```python
from build123d import *

# Parameters (mm, degrees)
SKETCH1_W           = 25
SKETCH1_H           = 5
SKETCH2_R           = 3.625
BOSS_EXTRUDE1_DEPTH = 3
CUT_EXTRUDE1_DEPTH  = 37.463627082
CUT_EXTRUDE2_DEPTH  = 36.924867432
CUT_EXTRUDE3_DEPTH  = 36.924867432
CUT_EXTRUDE4_DEPTH  = 36.924867432
CUT_EXTRUDE5_DEPTH  = 36.924867432
CUT_EXTRUDE6_DEPTH  = 36.924867432
CUT_EXTRUDE7_DEPTH  = 36.924867432
CUT_EXTRUDE8_DEPTH  = 36.924867432
CUT_EXTRUDE9_DEPTH  = 37.463627082


with BuildPart() as part:
    # Sketch1 → Revolve1 (revolve)
    with BuildSketch(Plane(origin=(0, 0, 0), x_dir=(1, 0, 0), z_dir=(0, 1, 0))):
        with Locations((12.19, 88.3)):
            Rectangle(SKETCH1_W, SKETCH1_H)
    revolve(axis=Axis((-0.31, 0, -90.8), (0, 0, 1)))

    # Sketch2 → Boss-Extrude1 (add)
    with BuildSketch(Plane.XY.offset(-85.8)):
        with Locations((-0.31, 0)):
            Circle(SKETCH2_R)
    extrude(amount=BOSS_EXTRUDE1_DEPTH)

    # Sketch3 → Cut-Extrude1 (cut, through all)
    with BuildSketch(Plane(origin=(0, 0, -90.8), x_dir=(-1, 0, 0), z_dir=(0, 0, -1))):
        with BuildLine():
            Line((-1.738954013, -1.834199404), (2.358954013, -1.834199404))
            ThreePointArc((2.358954013, -1.834199404), (3.06, 0), (2.358954013, 1.834199404))
            Line((2.358954013, 1.834199404), (-1.738954013, 1.834199404))
            ThreePointArc((-1.738954013, 1.834199404), (-2.44, 0), (-1.738954013, -1.834199404))
        make_face()
    extrude(amount=-CUT_EXTRUDE1_DEPTH, mode=Mode.SUBTRACT)

    # Sketch4 → Cut-Extrude2 (cut, through all)
    with BuildSketch(Plane.XY.offset(-85.8)):
        with BuildLine():
            Line((5.725533906, 1), (15.382388155, 1))
            ThreePointArc((15.382388155, 1), (20.463725584, 8.604758878), (11.493300859, 10.389087297))
            Line((11.493300859, 10.389087297), (4.664873734, 3.560660172))
            ThreePointArc((4.664873734, 3.560660172), (4.339714607, 1.925974851), (5.725533906, 1))
        make_face()
    extrude(amount=-CUT_EXTRUDE2_DEPTH, mode=Mode.SUBTRACT)

    # Sketch5 → Cut-Extrude3 (cut, through all)
    with BuildSketch(Plane.XY.offset(-85.8)):
        with BuildLine():
            Line((-12.113300859, -10.389087297), (-5.284873734, -3.560660172))
            ThreePointArc((-5.284873734, -3.560660172), (-4.959714607, -1.925974851), (-6.345533906, -1))
            Line((-6.345533906, -1), (-16.002388155, -1))
            ThreePointArc((-16.002388155, -1), (-21.083725584, -8.604758878), (-12.113300859, -10.389087297))
        make_face()
    extrude(amount=-CUT_EXTRUDE3_DEPTH, mode=Mode.SUBTRACT)

    # Sketch6 → Cut-Extrude4 (cut, through all)
    with BuildSketch(Plane.XY.offset(-85.8)):
        with BuildLine():
            Line((3.250660172, 4.974873734), (10.079087297, 11.803300859))
            ThreePointArc((10.079087297, 11.803300859), (8.294758878, 20.773725584), (0.69, 15.692388155))
            Line((0.69, 15.692388155), (0.69, 6.035533906))
            ThreePointArc((0.69, 6.035533906), (1.615974851, 4.649714607), (3.250660172, 4.974873734))
        make_face()
    extrude(amount=-CUT_EXTRUDE4_DEPTH, mode=Mode.SUBTRACT)

    # Sketch7 → Cut-Extrude5 (cut, through all)
    with BuildSketch(Plane.XY.offset(-85.8)):
        with BuildLine():
            Line((-3.870660172, -4.974873734), (-10.699087297, -11.803300859))
            ThreePointArc((-10.699087297, -11.803300859), (-8.914758878, -20.773725584), (-1.31, -15.692388155))
            Line((-1.31, -15.692388155), (-1.31, -6.035533906))
            ThreePointArc((-1.31, -6.035533906), (-2.235974851, -4.649714607), (-3.870660172, -4.974873734))
        make_face()
    extrude(amount=-CUT_EXTRUDE5_DEPTH, mode=Mode.SUBTRACT)

    # Sketch8 → Cut-Extrude6 (cut, through all)
    with BuildSketch(Plane.XY.offset(-85.8)):
        with BuildLine():
            Line((15.382388155, -1), (5.725533906, -1))
            ThreePointArc((5.725533906, -1), (4.339714607, -1.925974851), (4.664873734, -3.560660172))
            Line((4.664873734, -3.560660172), (11.493300859, -10.389087297))
            ThreePointArc((11.493300859, -10.389087297), (20.463725584, -8.604758878), (15.382388155, -1))
        make_face()
    extrude(amount=-CUT_EXTRUDE6_DEPTH, mode=Mode.SUBTRACT)

    # Sketch9 → Cut-Extrude7 (cut, through all)
    with BuildSketch(Plane.XY.offset(-85.8)):
        with BuildLine():
            Line((-16.002388155, 1), (-6.345533906, 1))
            ThreePointArc((-6.345533906, 1), (-4.959714607, 1.925974851), (-5.284873734, 3.560660172))
            Line((-5.284873734, 3.560660172), (-12.113300859, 10.389087297))
            ThreePointArc((-12.113300859, 10.389087297), (-21.083725584, 8.604758878), (-16.002388155, 1))
        make_face()
    extrude(amount=-CUT_EXTRUDE7_DEPTH, mode=Mode.SUBTRACT)

    # Sketch10 → Cut-Extrude8 (cut, through all)
    with BuildSketch(Plane.XY.offset(-85.8)):
        with BuildLine():
            Line((-1.31, 6.035533906), (-1.31, 15.692388155))
            ThreePointArc((-1.31, 15.692388155), (-8.914758878, 20.773725584), (-10.699087297, 11.803300859))
            Line((-10.699087297, 11.803300859), (-3.870660172, 4.974873734))
            ThreePointArc((-3.870660172, 4.974873734), (-2.235974851, 4.649714607), (-1.31, 6.035533906))
        make_face()
    extrude(amount=-CUT_EXTRUDE8_DEPTH, mode=Mode.SUBTRACT)

    # Sketch11 → Cut-Extrude9 (cut, through all)
    with BuildSketch(Plane(origin=(0, 0, -90.8), x_dir=(-1, 0, 0), z_dir=(0, 0, -1))):
        with BuildLine():
            Line((-0.69, -15.692388155), (-0.69, -6.035533906))
            ThreePointArc((-0.69, -6.035533906), (-1.615974851, -4.649714607), (-3.250660172, -4.974873734))
            Line((-3.250660172, -4.974873734), (-10.079087297, -11.803300859))
            ThreePointArc((-10.079087297, -11.803300859), (-8.294758878, -20.773725584), (-0.69, -15.692388155))
        make_face()
    extrude(amount=-CUT_EXTRUDE9_DEPTH, mode=Mode.SUBTRACT)


solid = part.part
```
Could you check a few things on this model? Use its own coordinates, in mm. Round coordinates to 2 decimals unless told otherwise and drop trailing zeros. Loops run counter-clockwise (first coordinate to the right, second up) from the corner with the lowest first, then second, coordinate; pieces in that order, holes last. Notation, with made-up numbers: (84.5, -34.5) - (103.5, -34.5) arc R24 cw to (103.5, -14.5) - close; hole circle Ø8 at (33.5, 70). An arc over 180 degrees is marked (long way). Use CSV: the item, a comma, the result in double quotes.
Item 1: I need wall thicknesses on L1, parallel to Y at x = -20, z = -87.5; L2, parallel to Y at x = -6.81, z = -87.6; L3, parallel to X at y = 6.5, z = -87. Which ranges of each line are inside material? Lowest first, please. Write a range as [from, to].
Here are the results:
L1,"y = [-15.4, -10.28], [-2.72, 2.72], [10.28, 15.4]"
L2,"y = [-24.14, -21.19], [-7.91, -5.09], [-1, 1], [5.09, 7.91], [21.19, 24.14]"
L3,"x = [-24.45, -21.5], [-8.22, -5.4], [-1.31, 0.69], [4.78, 7.6], [20.88, 23.83]"
Item 2: If we section it at A-A on y = 0: List the corners of the cut face in (x, z) for me (3 decimals), then the cut area to 3 significant figures.
Here are the results:
outline,"(-25.31, -90.8) - (-3.06, -90.8) - (-3.06, -82.8) - (-3.935, -82.8) - (-3.935, -85.8) - (-25.31, -85.8) - close; (2.44, -90.8) - (24.69, -90.8) - (24.69, -85.8) - (3.315, -85.8) - (3.315, -82.8) - (2.44, -82.8) - close"
area,"228 mm²"
Item 3: If we section it at B-B on x = -0.31: List the corners of the cut face in (y, z) for me (3 decimals), then the cut area to 3 significant figures.
Here are the results:
outline,"(-25, -90.8) - (-1.834, -90.8) - (-1.834, -82.8) - (-3.625, -82.8) - (-3.625, -85.8) - (-25, -85.8) - close; (1.834, -90.8) - (25, -90.8) - (25, -85.8) - (3.625, -85.8) - (3.625, -82.8) - (1.834, -82.8) - close"
area,"242 mm²"
Item 4: If we mould it in two halves opening along Y, with no side actions, what happens to faces 1 (the cylindrical face through (23.536, 7.509, -88.335)), 2 (the flat face through (-6, 0, -90.8)), 3 (the flat face through (-11, -1, -88))? For each: pulls with the +Y half, pulls with the -Y half, needs draft (parallel to the pull), parting line crosses it, or undercut.
Here are the results:
face 1,"parting line crosses it"
face 2,"needs draft"
face 3,"undercut"
Item 5: Will these pins go through, and if not, where does the flat tip stop? pin 1 (4.5 mm diameter, centred on x = 0, z = -85.5, fed in from -Y); pin 2 (1.5 mm diameter, centred on x = -0.5, y = -17.5, fed in from +Z); pin 3 (1 mm diameter, centred on x = 2, z = -88, fed in from -Y).
Here are the results:
pin 1,"stops at y = -25"
pin 2,"stops at z = -85.8"
pin 3,"stops at y = -24.93"
Item 6: If we section it at C-C on z = -84.5: List the corners of the cut face in (x, y) for me (3 decimals), then the cut area to 3 significant figures.
Here are the results:
outline,"circle Ø7.25 at (-0.31, 0); hole (-2.359, -1.834) - (1.739, -1.834) arc R2.75 ccw to (1.739, 1.834) - (-2.359, 1.834) arc R2.75 ccw to start"
area,"22.7 mm²"
Item 7: If we section it at D-D on y = -17: List the corners of the cut face in (x, z) for me.
Here are the results:
outline,"(-18.64, -90.8) - (-12.15, -90.8) - (-12.15, -85.8) - (-18.64, -85.8) - close; (-1.47, -90.8) - (0.85, -90.8) - (0.85, -85.8) - (-1.47, -85.8) - close; (11.53, -90.8) - (18.02, -90.8) - (18.02, -85.8) - (11.53, -85.8) - close"
